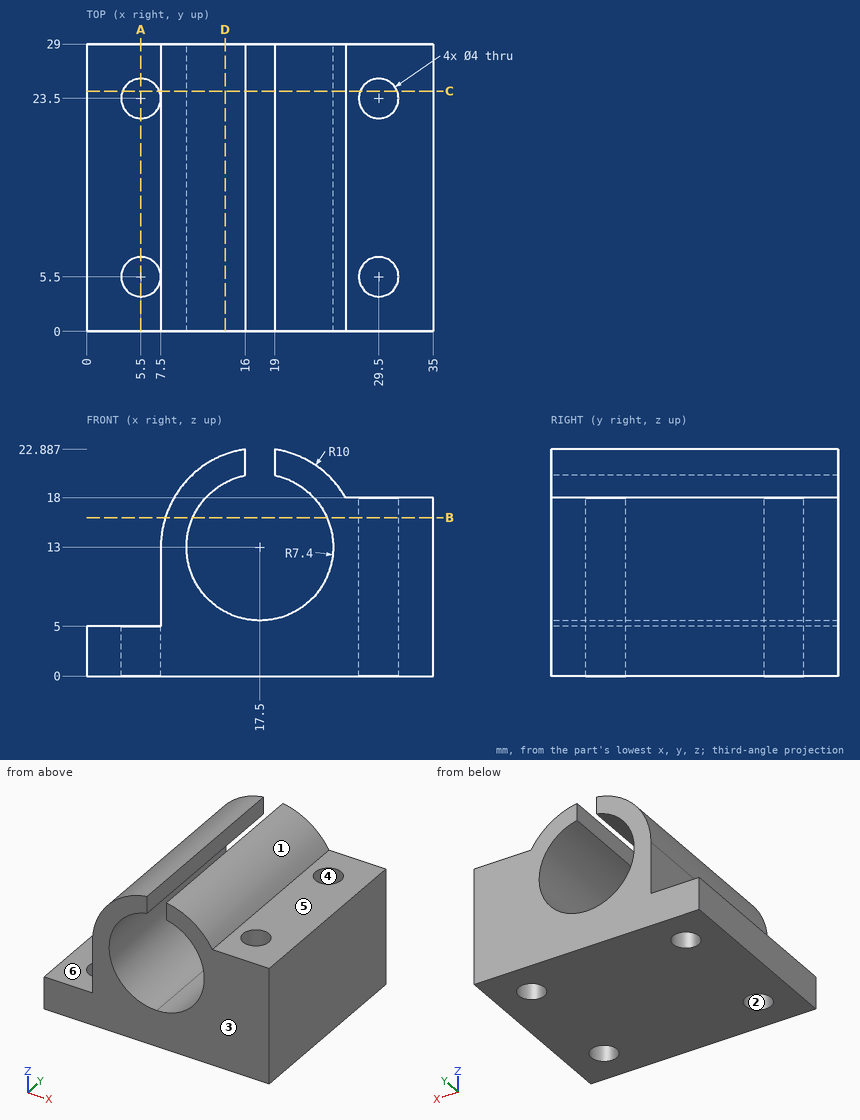
Part print with two shaded views. Sizes in mm from the minimum x, y, z corner. A direction names the side the tool comes from. Round coordinates to 2 decimals unless told otherwise and drop trailing zeros. Write each loop counter-clockwise with the first axis right and the second up, starting at its lowest first coordinate (ties: lowest second). Pieces come first, ordered by that corner, then holes. Notation, with made-up numbers: (-2.75, 13.25) -> (22.25, 13.25) arc R18 ccw to (22.25, 19.25) -> close; hole circle Ø7 at (65.25, 44.25). An arc over 180 degrees is marked (long way). Use one line per item in the form item = value.
Q1. Two-plate mould, pull along Y, no slides. Class the marked faces 1, 2 and 3: released by +Y, released by -Y, zero draft, split by the parting line, or undercut.
Conclusion:
face_1 = zero draft
face_2 = undercut
face_3 = released by -Y
Q2. Drop flat-ended pins along their axis: P1, Ø3, axis at y = 16, z = 21, coming from the +X side; P2, Ø5, axis at y = 10, z = 18, coming from the -X side; P3, Ø4, axis at y = 12, z = 10, coming from the -X side. Give the stop position or say it passes through.
Conclusion:
P1 = 25.1
P2 = 7.82
P3 = 7.5
Q3. Band-saw the part on D-D, the plane x = 14. Write the cut outline in (y, z).
Conclusion:
outline = (0, 0) -> (29, 0) -> (29, 6.48) -> (0, 6.48) -> close; (0, 19.52) -> (29, 19.52) -> (29, 22.37) -> (0, 22.37) -> close
Q4. Drill centre lines: L1, parallel to X at y = 23.5, z = 2.7; L2, parallel to Y at x = 5.5, z = 2.35; L3, parallel to X at y = 4.25, z = 17.75 (1 decimal). Where is each one in solid material? Low to high.
Conclusion:
L1 = 0 to 3.5, 7.5 to 27.5, 31.5 to 35
L2 = 0 to 3.5, 7.5 to 21.5, 25.5 to 29
L3 = 8.7 to 11.8, 23.2 to 27.9, 31.1 to 35
Q5. Band-saw the part on B-B, the plane z = 16. Write the cut outline in (x, y), then the cut area to 3 significant figures.
Conclusion:
outline = (7.96, 0) -> (10.74, 0) -> (10.74, 29) -> (7.96, 29) -> close; (24.26, 0) -> (35, 0) -> (35, 29) -> (24.26, 29) -> close; hole circle Ø4 at (29.5, 5.5); hole circle Ø4 at (29.5, 23.5)
area = 367 mm²
Q6. Band-saw the part on C-C, the plane y = 24.25. Write the cut outline in (x, z).
Conclusion:
outline = (0, 0) -> (3.65, 0) -> (3.65, 5) -> (0, 5) -> close; (7.35, 0) -> (27.65, 0) -> (27.65, 18) -> (26.16, 18) arc R10 ccw to (19, 22.89) -> (19, 20.25) arc R7.4 cw (long way) to (16, 20.25) -> (16, 22.89) arc R10 ccw to (7.5, 13) -> (7.5, 5) -> (7.35, 5) -> close; (31.35, 0) -> (35, 0) -> (35, 18) -> (31.35, 18) -> close
Q7. Band-saw the part on A-A, the plane x = 5.5. Write the cut outline in (y, z), then the cut area to 3 significant figures.
Conclusion:
outline = (0, 0) -> (3.5, 0) -> (3.5, 5) -> (0, 5) -> close; (7.5, 0) -> (21.5, 0) -> (21.5, 5) -> (7.5, 5) -> close; (25.5, 0) -> (29, 0) -> (29, 5) -> (25.5, 5) -> close
area = 105 mm²
Q8. Tool access for the marked faces 4, 5 and 6: list every direction of +Z, -Z, +X, -X, +Y, -Y with a clear straight run to the whole face (end or side of a thin tool).
Conclusion:
face_4 = +Z, -Z
face_5 = +Z, +X, +Y, -Y
face_6 = +Z, -X, +Y, -Y
